Could you check a few things on this model? Use its own coordinates, in mm. Give positions to 0.01 mm unless a question says otherwise; leave off trailing zeros. Order: outer loops, then holes, each group sorted by start corner. A loop starts at its lowest first (then second) coordinate and runs counter-clockwise, first axis right, second up. Notation, with made-up numbers: M -7,83 L 42,83 A26 ccw 42,122 Z; hole C 45.5,37.25 d2. An arc over 180 degrees is marked long. Use a Markdown table: item, result. Add a question column.
Item 1: If I drill on L1, parallel to Y at x = 0, z = 43.5; L2, parallel to Z at x = 7.5, y = 16.5, over which ranges is the centre line in solid material (lowest first)? Write a range as from..to.
Item 2: Suppose I cut it at A-A on z = 49.5. Write out the boundary of the cut face in (x, y), plus the area to 3 significant figures.
Item 3: Suppose I cut it at B-B on z = 18. Write out the boundary of the cut face in (x, y), plus the area to 3 significant figures.
Item 4: If we mould it in two halves opening along Z, with no side actions, what happens to faces 1 (the face through (0, 0, 0)), 2 (the face through (-0.194, 0.872, 3.445)), 3 (the face through (17.623, -5.55, 16.81)), 4 (the face through (6.888, 13.244, 45.829))? For each: released by +Z, released by -Z, zero draft, split by the parting line, or undercut.
Item 5: I'm going to push flat-ended pins straight in: pin 1 Ø12 at (x, z) = (15.5, 12) entering from -Y; pin 2 Ø8 at (x, z) = (-12, 46) entering from +Y; pin 3 Ø10 at (y, z) = (-2, 38.5) entering from -X. Where does each tip first touch, or does it pass through?
from build123d import *


# Not quite as in the source:
# - a fillet or chamfer that OpenCascade refuses, or shapes differently, is made with other operations: its cross-section is extruded or revolved along the edge and cut away or added


with BuildPart() as f1:
    # F0 (on Front) → F1 (revolve)
    with BuildSketch(Plane.XZ):
        with BuildLine():
            Line((0, 3.4511274384), (0, 0))
            Line((0, 0), (18.3868259192, 0))
            ThreePointArc((18.3868259192, 0), (20.9391502019, 1.1918933999), (21.6636881232, 3.9140274748))
            Line((21.6636881232, 3.9140274748), (21.6636881232, 30.6750517339))
            ThreePointArc((21.6636881232, 30.6750517339), (20.8362073086, 33.8137273466), (18.5688734055, 36.1364856362))
            Line((18.5688734055, 36.1364856362), (18.5688734055, 55.7976476848))
            Line((18.5688734055, 55.7976476848), (14.9279180914, 55.7976476848))
            Line((14.9279180914, 55.7976476848), (14.9279180914, 36.1364856362))
            ThreePointArc((14.9279180914, 36.1364856362), (17.4559954455, 33.877501736), (18.5688734055, 30.6750517339))
            Line((18.5688734055, 30.6750517339), (18.3868259192, 3.3287243314))
            Line((18.3868259192, 3.3287243314), (0, 3.4511274384))
        make_face()
    revolve(axis=Axis((0, 0, 1.7255637192), (0, 0, -1)))

    # F2: fillet of radius 5.08 on 1 edges, made by hand

    # F2_s1 → F2_t2 (revolve, cut)
    with BuildSketch(Plane.XZ):
        with BuildLine():
            ThreePointArc((18.5688734055, 50.9257332365), (17.5580715454, 53.9667900425), (14.9279180914, 55.7976476848))
            Line((14.9279180914, 55.7976476848), (18.5688734055, 55.7976476848))
            Line((18.5688734055, 55.7976476848), (18.5688734055, 50.9257332365))
        make_face()
    revolve(axis=Axis((0, 0, 55.7976476848), (0, 0, -1)), mode=Mode.SUBTRACT)


solid = f1.part
Findings below:
| question | item | result |
|---|---|---|
| 1 | L1 | y = -18.57..-14.93, 14.93..18.57 |
| 1 | L2 | z = 0..3.33, 32.6..53 |
| 2 | outline | C 0,0 d37.14; hole C 0,0 d29.86 |
| 2 | area | 383 mm^2 |
| 3 | outline | C 0,0 d43.33; hole C 0,0 d36.97 |
| 3 | area | 401 mm^2 |
| 4 | face 1 | released by -Z |
| 4 | face 2 | undercut |
| 4 | face 3 | undercut |
| 4 | face 4 | zero draft |
| 5 | pin 1 | stops at y = -19.47 |
| 5 | pin 2 | stops at y = 16.76 |
| 5 | pin 3 | stops at x = -20.94 |
